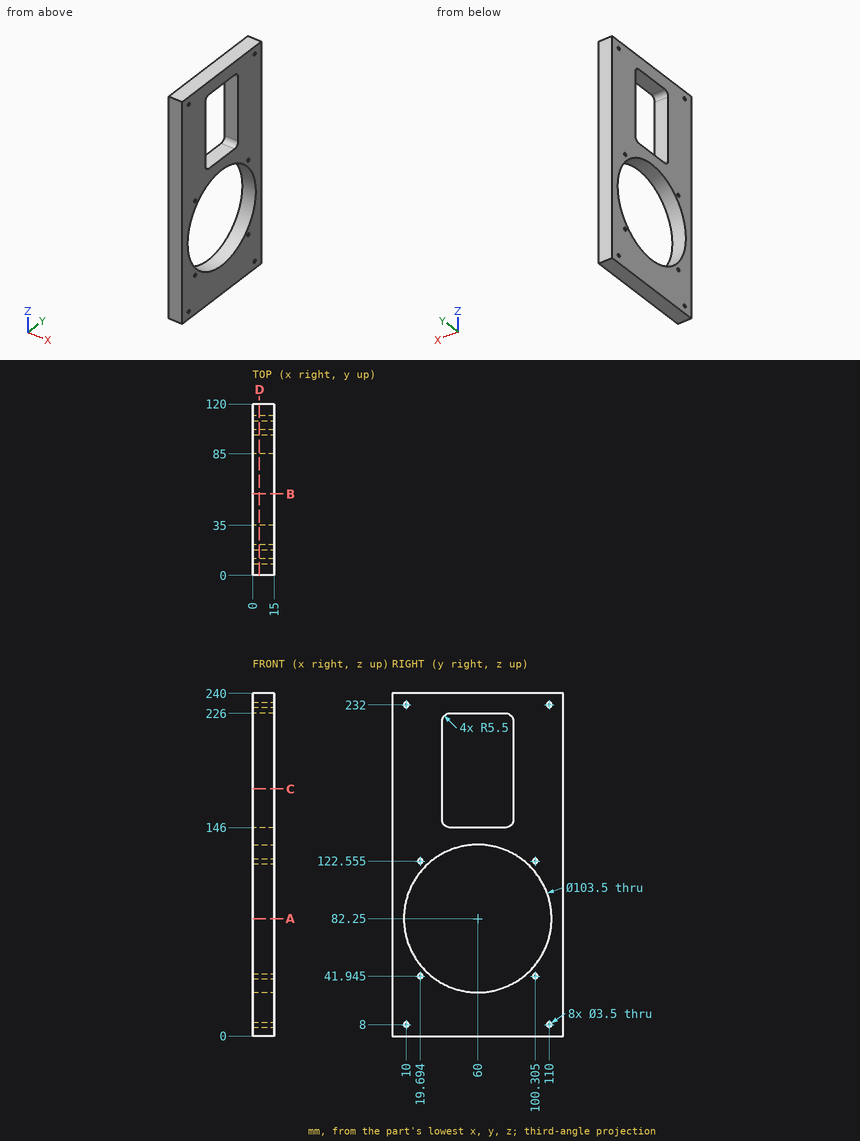
Geometry: see drawing. Coordinates: mm, zero at the bounding-box minimum. Coordinates: 2 decimals unless noted, no trailing zeros. Write each loop counter-clockwise with the first axis right and the second up, starting at its lowest first coordinate (ties: lowest second). Pieces come first, ordered by that corner, then holes.
1) Section C-C on z = 173. Output: boundary loops of the cut face in (x, y).
2) Section A-A on z = 82.25. Output: boundary loops of the cut face in (x, y).
3) Section B-B on y = 57. Output: boundary loops of the cut face in (x, z), and give its area (3 significant figures).
4) Section D-D on x = 4.75. State how many separate pieces and enclosed holes the cut face has, and give its area (3 significant figures).
5) Material intervals for line 1 along Z through (x, y) = (7.75, 60); line 2 along Y through (x, z) = (4.75, 8); line 3 along Y through (x, z) = (10.25, 209.5), sorted ascending.
Check result:
1. outline: (0, 0) - (15, 0) - (15, 35) - (0, 35) - close; (0, 85) - (15, 85) - (15, 120) - (0, 120) - close
2. outline: (0, 0) - (15, 0) - (15, 8.25) - (0, 8.25) - close; (0, 111.75) - (15, 111.75) - (15, 120) - (0, 120) - close
3. outline: (0, 0) - (15, 0) - (15, 30.59) - (0, 30.59) - close; (0, 133.91) - (15, 133.91) - (15, 146) - (0, 146) - close; (0, 226) - (15, 226) - (15, 240) - (0, 240) - close
3. area: 850 mm2
4. separate pieces: 1
4. enclosed holes: 10
4. area: 16,300 mm2
5. line 1: z = 0 to 30.5, 134 to 146, 226 to 240
5. line 2: y = 0 to 8.25, 11.75 to 108.25, 111.75 to 120
5. line 3: y = 0 to 35, 85 to 120
